```python
from build123d import *

# Parameters (mm, degrees)
OTHER_10076_5_DEPTH = 0.5
CUT_EXTRUDE1_START  = -0.5
CUT_EXTRUDE1_DEPTH  = 0.5


# Read off the part's stored shape, not the designer's step: 10076-5
with BuildPart() as part:
    # Other 10076-5 outline → Other 10076-5 (new body)
    with BuildSketch(Plane.XY):
        with BuildLine():
            ThreePointArc((7.573674013, -9.436602245), (7.668819519, -9.359444812), (7.763179028, -9.281328104))
            Line((7.763179028, -9.281328104), (7.919995926, -7.488902759))
            ThreePointArc((7.919995926, -7.488902759), (8.548470738, -6.76266575), (9.110578105, -5.983925684))
            ThreePointArc((9.110578105, -5.983925684), (9.242448569, -5.182849851), (8.736493865, -4.547930843))
            Line((8.736493865, -4.547930843), (8.260223146, -4.3))
            Line((8.260223146, -4.3), (5.774945887, -4.3))
            ThreePointArc((5.774945887, -4.3), (5.659072475, -4.451392897), (5.53923133, -4.5996648))
            Line((5.53923133, -4.5996648), (6.59, -6.419649523))
            ThreePointArc((6.59, -6.419649523), (5.831509763, -7.1157216), (5, -7.722693831))
            Line((5, -7.722693831), (5, -7.841555968))
            ThreePointArc((5, -7.841555968), (0, -9.3), (-5, -7.841555968))
            Line((-5, -7.841555968), (-5, -7.722693831))
            ThreePointArc((-5, -7.722693831), (-5.831509763, -7.1157216), (-6.59, -6.419649523))
            Line((-6.59, -6.419649523), (-5.53923133, -4.5996648))
            ThreePointArc((-5.53923133, -4.5996648), (-5.659072475, -4.451392897), (-5.774945887, -4.3))
            Line((-5.774945887, -4.3), (-8.260223146, -4.3))
            Line((-8.260223146, -4.3), (-10.732831081, -5.58715822))
            ThreePointArc((-10.732831081, -5.58715822), (-10.675718173, -5.6955282), (-10.617511084, -5.803314431))
            Line((-10.617511084, -5.803314431), (-9.055174855, -6.258693914))
            ThreePointArc((-9.055174855, -6.258693914), (-8.704696722, -6.64117368), (-8.882127626, -7.128661083))
            Line((-8.882127626, -7.128661083), (-9.436602245, -7.573674013))
            ThreePointArc((-9.436602245, -7.573674013), (-9.359444812, -7.668819519), (-9.281328104, -7.763179028))
            Line((-9.281328104, -7.763179028), (-7.660171598, -7.905011844))
            ThreePointArc((-7.660171598, -7.905011844), (-7.241809703, -8.211767477), (-7.320727248, -8.724502998))
            Line((-7.320727248, -8.724502998), (-7.777730077, -9.269137762))
            ThreePointArc((-7.777730077, -9.269137762), (-7.683493234, -9.347402405), (-7.588468891, -9.424709008))
            Line((-7.588468891, -9.424709008), (-5.970792243, -9.247544602))
            ThreePointArc((-5.970792243, -9.247544602), (-5.500623999, -9.466787654), (-5.477995427, -9.985067155))
            Line((-5.477995427, -9.985067155), (-5.819964104, -10.608393744))
            ThreePointArc((-5.819964104, -10.608393744), (-5.712269322, -10.666769858), (-5.603989074, -10.724052707))
            Line((-5.603989074, -10.724052707), (-4.05195869, -10.234699407))
            ThreePointArc((-4.05195869, -10.234699407), (-3.548052399, -10.358004491), (-3.424747314, -10.861910782))
            Line((-3.424747314, -10.861910782), (-3.638540174, -11.539975104))
            ThreePointArc((-3.638540174, -11.539975104), (-3.521526102, -11.576219327), (-3.404151099, -11.611277074))
            Line((-3.404151099, -11.611277074), (-1.977410637, -10.828540453))
            ThreePointArc((-1.977410637, -10.828540453), (-1.459131136, -10.851169025), (-1.239888083, -11.321337268))
            Line((-1.239888083, -11.321337268), (-1.317289186, -12.028081692))
            ThreePointArc((-1.317289186, -12.028081692), (-1.195452609, -12.04080118), (-1.073493507, -12.052286575))
            Line((-1.073493507, -12.052286575), (0.173128198, -11.006246762))
            ThreePointArc((0.173128198, -11.006246762), (0.685863719, -10.927329218), (0.992619352, -11.345691113))
            Line((0.992619352, -11.345691113), (1.054584487, -12.053955847))
            ThreePointArc((1.054584487, -12.053955847), (1.176561457, -12.042661796), (1.298417839, -12.030133462))
            Line((1.298417839, -12.030133462), (2.317013814, -10.760989181))
            ThreePointArc((2.317013814, -10.760989181), (2.804501216, -10.583558277), (3.186980982, -10.93403641))
            Line((3.186980982, -10.93403641), (3.38593107, -11.616603238))
            ThreePointArc((3.38593107, -11.616603238), (3.503360927, -11.581729673), (3.620431715, -11.545669067))
            Line((3.620431715, -11.545669067), (4.371857887, -10.10219282))
            ThreePointArc((4.371857887, -10.10219282), (4.815363304, -9.833067127), (5.258868721, -10.10219282))
            Line((5.258868721, -10.10219282), (5.58715822, -10.732831081))
            ThreePointArc((5.58715822, -10.732831081), (5.6955282, -10.675718173), (5.803314431, -10.617511084))
            Line((5.803314431, -10.617511084), (6.258693914, -9.055174855))
            ThreePointArc((6.258693914, -9.055174855), (6.64117368, -8.704696722), (7.128661083, -8.882127626))
            Line((7.128661083, -8.882127626), (7.573674013, -9.436602245))
        make_face()
    extrude(amount=OTHER_10076_5_DEPTH)

    # Sketch1 → Cut-Extrude1 (cut)
    with BuildSketch(Plane.XY.offset(0.5).offset(CUT_EXTRUDE1_START)):
        with BuildLine():
            Line((-9.668418082, -5.033059884), (-10.732831081, -5.58715822))
            ThreePointArc((-10.732831081, -5.58715822), (-4.639236905, -11.175306749), (3.620431715, -11.545669067))
            Line((3.620431715, -11.545669067), (4.371857887, -10.10219282))
            ThreePointArc((4.371857887, -10.10219282), (4.469650209, -9.971843573), (4.604163159, -9.879862428))
            ThreePointArc((4.604163159, -9.879862428), (-3.50493127, -10.321117032), (-9.668418082, -5.033059884))
        make_face()
        with BuildLine():
            Line((7.573674013, -9.436602245), (7.128661083, -8.882127626))
            ThreePointArc((7.128661083, -8.882127626), (6.804041546, -8.699374782), (6.443160998, -8.791795969))
            ThreePointArc((6.443160998, -8.791795969), (7.211064546, -8.173771964), (7.919995926, -7.488902759))
            Line((7.919995926, -7.488902759), (7.763179028, -9.281328104))
            ThreePointArc((7.763179028, -9.281328104), (7.668819519, -9.359444812), (7.573674013, -9.436602245))
        make_face()
    extrude(amount=CUT_EXTRUDE1_DEPTH, mode=Mode.SUBTRACT)


solid = part.part
```
Geometry check sheet. Reference: the model listing, model coordinates, mm. A direction names the side the tool comes from. Coordinates: 2 decimals unless noted, no trailing zeros. Loops run counter-clockwise (first coordinate to the right, second up) from the corner with the lowest first, then second, coordinate; pieces in that order, holes last.
Item 1: Release check for a two-part mould opening along Y. For faces 3 (the face through (-5.82, -7.125, 0.246)), 4 (the face through (-6.07, -5.52, 0.25)), 5 (the face through (-3.39, -10.36, 0.25)), 6 (the face through (0, -10, 0)) record: released by +Y, released by -Y, zero draft, split by the parting line, or undercut.
Item 2: Sectioned sample at A-A, the plane x = 6. Record the boundary of the cut face in (y, z), then the cut area to 3 significant figures.
Item 3: Access from +Z, -Z, +X, -X, +Y, -Y to the whole of each face (thin tool, end or side, straight path). Record for faces 1 (the face through (0.1, -9.3, 0.2)), 2 (the face through (5.84, -7.11, 0.25)).
Item 4: Thickness scan on line 1 (X direction, y = -8.25, z = 0.25); line 2 (X direction, y = -7.75, z = 0.2); line 3 (Y direction, x = -6.25, z = 0.35). Record the ranges inside material, lowest first.
Item 5: Sectioned sample at D-D, the plane x = -7. Record the boundary of the cut face in (y, z), then the cut area to 3 significant figures.
Item 6: Sectioned sample at C-C, the plane z = 0.15. Record the boundary of the cut face in (x, y).
Item 7: Sectioned sample at B-B, the plane y = -5.75. Record the boundary of the cut face in (x, z), then the cut area to 3 significant figures.
Check result:
1. face 3: undercut
1. face 4: undercut
1. face 5: released by -Y
1. face 6: zero draft
2. outline: (-9.94, 0) - (-6.97, 0) - (-6.97, 0.5) - (-9.94, 0.5) - close; (-5.4, 0) - (-4.3, 0) - (-4.3, 0.5) - (-5.4, 0.5) - close
2. area: 2.03 mm2
3. face 1: +Z, -Z, +Y
3. face 2: +Z, -Z
4. line 1: x = -7.12 to -4.29, 4.29 to 7.12
4. line 2: x = -7.66 to -5, 5 to 7.66
4. line 3: y = -8.93 to -6.75, -5.83 to -4.3
5. outline: (-8.36, 0) - (-4.3, 0) - (-4.3, 0.5) - (-8.36, 0.5) - close
5. area: 2.03 mm2
6. outline: (-9.67, -5.03) arc R10.9 ccw to (4.6, -9.88) arc R0.5 cw to (5.26, -10.1) - (5.59, -10.73) arc R12.1 ccw to (5.8, -10.62) - (6.26, -9.06) arc R0.5 cw to (6.44, -8.79) arc R10.9 ccw to (9.11, -5.98) arc R1 ccw to (8.74, -4.55) - (8.26, -4.3) - (5.77, -4.3) arc R7.2 cw to (5.54, -4.6) - (6.59, -6.42) arc R9.2 cw to (5, -7.72) - (5, -7.84) arc R9.3 cw to (-5, -7.84) - (-5, -7.72) arc R9.2 cw to (-6.59, -6.42) - (-5.54, -4.6) arc R7.2 cw to (-5.77, -4.3) - (-8.26, -4.3) - close
7. outline: (-9.26, 0) - (-6.2, 0) - (-6.2, 0.5) - (-9.26, 0.5) - close; (6.2, 0) - (9.22, 0) - (9.22, 0.5) - (6.2, 0.5) - close
7. area: 3.04 mm2
